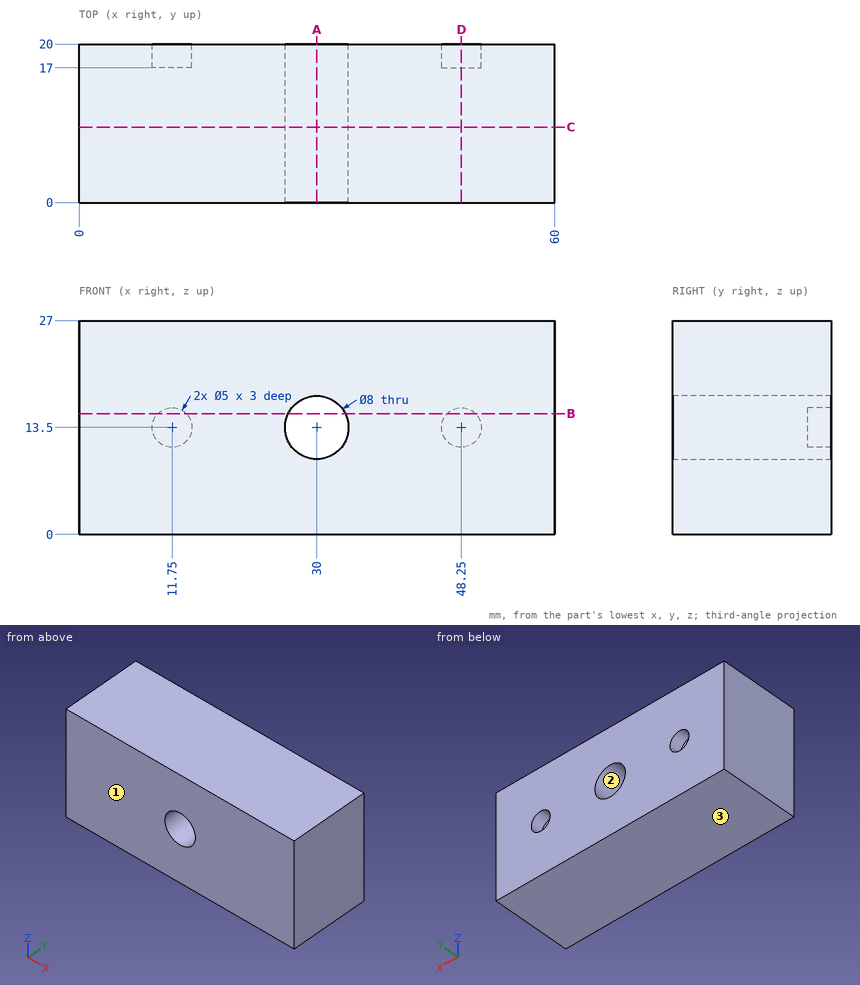
Source: three-view drawing plus pictorial views. Frame: mm from the lowest corner of the part. Round coordinates to 2 decimals unless told otherwise and drop trailing zeros. Order: outer loops, then holes, each group sorted by start corner. A loop starts at its lowest first (then second) coordinate and runs counter-clockwise, first axis right, second up. Notation, with made-up numbers: (77.5, 14) - (118.5, 14) arc R35 cw to (118.5, 50) - close; hole circle Ø1 at (16, -14.5). An arc over 180 degrees is marked (long way). Answer in a Markdown table with one row per item.
Item 1: Section query A-A (x = 30). Return the cut outline in (y, z), then the cut area to 3 significant figures.
Model answer:
| item | result |
|---|---|
| outline | (0, 0) - (20, 0) - (20, 9.5) - (0, 9.5) - close; (0, 17.5) - (20, 17.5) - (20, 27) - (0, 27) - close |
| area | 380 mm² |
Item 2: Mould query, pull axis Z, two halves, no side actions, for the marked faces 1, 2 and 3. Classes: released by +Z, released by -Z, zero draft, split by the parting line, or undercut.
Model answer:
| item | result |
|---|---|
| face 1 | zero draft |
| face 2 | undercut |
| face 3 | released by -Z |
Item 3: Section query C-C (y = 9.5). Return the cut outline in (x, z).
Model answer:
| item | result |
|---|---|
| outline | (0, 0) - (60, 0) - (60, 27) - (0, 27) - close; hole circle Ø8 at (30, 13.5) |
Item 4: Section query D-D (x = 48.25). Return the cut outline in (y, z), then the cut area to 3 significant figures.
Model answer:
| item | result |
|---|---|
| outline | (0, 0) - (20, 0) - (20, 11) - (17, 11) - (17, 16) - (20, 16) - (20, 27) - (0, 27) - close |
| area | 525 mm² |
Item 5: Section query B-B (z = 15.25). Return the cut outline in (x, y), then the cut area to 3 significant figures.
Model answer:
| item | result |
|---|---|
| outline | (0, 0) - (26.4, 0) - (26.4, 20) - (13.54, 20) - (13.54, 17) - (9.96, 17) - (9.96, 20) - (0, 20) - close; (33.6, 0) - (60, 0) - (60, 20) - (50.04, 20) - (50.04, 17) - (46.46, 17) - (46.46, 20) - (33.6, 20) - close |
| area | 1,030 mm² |
Item 6: Line query: line 1 (Z direction, x = 48.25, y = 18.15); line 2 (X direction, y = 19.05, z = 13.5); line 3 (X direction, y = 15.5, z = 13.25). Output: solid intervals per line, ascending.
Model answer:
| item | result |
|---|---|
| line 1 | z = 0 to 11, 16 to 27 |
| line 2 | x = 0 to 9.25, 14.25 to 26, 34 to 45.75, 50.75 to 60 |
| line 3 | x = 0 to 26.01, 33.99 to 60 |
Item 7: Pin query (flat end, axial travel): pin 1 (4 mm diameter, centred on x = 48.25, z = 13.5, fed in from +Y). Return the tip coordinate at first contact, or that it passes through.
Model answer:
| item | result |
|---|---|
| pin 1 | stops at y = 17 |
